from build123d import *

# Parameters (mm, degrees)
SKETCH1_W           = 101.6
SKETCH1_H           = 101.6
BOSS_EXTRUDE1_DEPTH = 98.425
SKETCH2_R           = 44.45
CUT_EXTRUDE1_DEPTH  = 69.85
SKETCH3_R           = 10.16
CUT_EXTRUDE2_DEPTH  = 25.4
FILLET1_R           = 50.8


with BuildPart() as part:
    # Sketch1 → Boss-Extrude1 (new body)
    with BuildSketch(Plane(origin=(0, 0, 0), x_dir=(1, 0, 0), z_dir=(0, 1, 0))):
        with Locations((50.8, -50.8)):
            Rectangle(SKETCH1_W, SKETCH1_H)
    extrude(amount=BOSS_EXTRUDE1_DEPTH)

    # Sketch2 → Cut-Extrude1 (cut)
    with BuildSketch(Plane(origin=(0, 98.425, 0), x_dir=(1, 0, 0), z_dir=(0, 1, 0))):
        with Locations(Location((50.8, -50.8, 0), (0, 0, 270))):
            Circle(SKETCH2_R)
    extrude(amount=-CUT_EXTRUDE1_DEPTH, mode=Mode.SUBTRACT)

    # Sketch3 → Cut-Extrude2 (cut)
    with BuildSketch(Plane(origin=(0, 28.575, 0), x_dir=(1, 0, 0), z_dir=(0, 1, 0))):
        with Locations(Location((63.631609733, -73.025, 0), (0, 0, 270))):
            Circle(SKETCH3_R)
        with Locations(Location((25.136780535, -50.8, 0), (0, 0, 270))):
            Circle(SKETCH3_R)
        with Locations(Location((63.631609733, -28.575, 0), (0, 0, 270))):
            Circle(SKETCH3_R)
    extrude(amount=-CUT_EXTRUDE2_DEPTH, mode=Mode.SUBTRACT)

    # Fillet1
    fillet1_edges = [part.edges().sort_by_distance(p)[0] for p in [
        (0, 49.2125, 101.6),
        (0, 49.2125, 0),
        (101.6, 49.2125, 0),
        (101.6, 49.2125, 101.6),
    ]]
    fillet(fillet1_edges, radius=FILLET1_R - 0.0001)  # a hair under: the kernel refuses the full size


solid = part.part
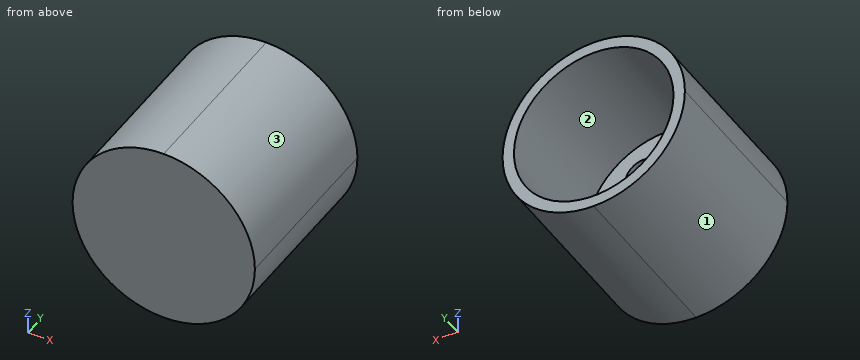
Read the model definition and answer for the solid it produces. Units are mm, in the model's axes. Face numbers are marked on the shaded views. Coordinates: 2 decimals unless noted, no trailing zeros. Order: outer loops, then holes, each group sorted by start corner. A loop starts at its lowest first (then second) coordinate and runs counter-clockwise, first axis right, second up. Notation, with made-up numbers: M -22,-28 L 10,-28 A32 ccw 10,9 Z; hole C 76,80.25 d4. An arc over 180 degrees is marked long. Put each result on its own line as item: value. Start each with the question number.
Item 1: Consider probe 1 along Y at (x, z) = (41.5, 42) (3 decimals); probe 2 along X at (y, z) = (67.5, 33.5); probe 3 along Z at (x, y) = (77, 76). Determine where each line is inside the solid, lowest interval first. Write a range as [from, to].
Item 2: Section D-D, the plane y = 14 is taken. Count the separate pieces of the cut face and the enclosed holes in it, plus the area to 3 significant figures.
Item 3: The mould has two halves that part along X. Classify the marked faces 1, 2 and 3: +X half, -X half, draft (parallel to the pull), parting line (faces both ways), or undercut.
Item 4: Given pin 1 Ø4 at (x, y) = (66.5, 86) entering from +Z; pin 2 Ø1.5 at (x, y) = (15, 27) entering from -Z; pin 3 Ø22.5 at (x, z) = (60.5, 72) entering from +Y (3 decimals), each flat-ended and moving along its own axis, determine where each tip first touches the part or whether it passes through.
Item 5: Section C-C, the plane x = 23 is taken. Determine the outline of the cut face in (y, z) (3 decimals), plus the area to 3 significant figures.
Item 6: Section B-B, the plane z = 13 is taken. Determine the outline of the cut face in (x, y) (3 decimals), plus the area to 3 significant figures.
Computed:
1. probe 1: y = [0, 28.575]
1. probe 2: x = [3.04, 9.85], [91.75, 98.56]
1. probe 3: z = [7.28, 14.89], [86.71, 94.32]
2. separate pieces: 1
2. enclosed holes: 3
2. area: 7,130 mm2
3. face 1: -X half
3. face 2: undercut
3. face 3: +X half
4. pin 1: stops at z = 99.72
4. pin 2: stops at z = 14.03
4. pin 3: stops at y = 28.575
5. outline: M 0,8.282 L 98.425,8.282 L 98.425,16.116 L 28.575,16.116 L 28.575,40.867 L 3.175,40.867 L 3.175,60.733 L 28.575,60.733 L 28.575,85.484 L 98.425,85.484 L 98.425,93.318 L 0,93.318 Z
5. area: 3,020 mm2
6. outline: M 16.862,0 L 84.738,0 L 84.738,98.425 L 74.187,98.425 L 74.187,28.575 L 27.413,28.575 L 27.413,98.425 L 16.862,98.425 Z
6. area: 3,410 mm2
